Model file for the job. Use its own axes, mm. A direction names the side the tool comes from. Give positions to 0.01 mm unless a question says otherwise; leave off trailing zeros. Loops run counter-clockwise (first coordinate to the right, second up) from the corner with the lowest first, then second, coordinate; pieces in that order, holes last. Notation, with made-up numbers: (87, 80.5) - (109, 80.5) arc R32 ccw to (109, 117.5) - close; hole circle Ø1 at (60, 60). An arc over 180 degrees is marked (long way). Answer as CSV lines item,"result". Start each with the question number.
Item 1: Drill centre lines: L1, parallel to X at y = 8.5, z = 0; L2, parallel to X at y = -18, z = 0; L3, parallel to Z at x = 25, y = 5.5. Where is each one in solid material? Low to high. Write a range as from..to.
Item 2: Saw through at B-B on x = 44. Give the cut face in (y, z).
Item 3: Saw through at D-D on y = 24. Give the cut face in (x, z), plus the area to 3 significant figures.
Item 4: Saw through at C-C on z = 39.5. Give the cut face in (x, y).
Item 5: Pull direction Y, two halves, no side cores. Call faces 5 (the conical face through (-31.429, 39.806, -6.979)), 6 (the cylindrical face through (-19.297, 8.112, 35.157)), 7 (the flat face through (0, 0, 0)), 8 (the flat face through (-23, 16, 23)): pulls with the +Y half, pulls with the -Y half, needs draft (parallel to the pull), parting line crosses it, or undercut.
Item 6: Pin check, flat tips, straight feed: pin 1 (1 mm diameter, centred on x = 40, z = 3, fed in from -Y); pin 2 (9 mm diameter, centred on x = -22, z = 38.11, fed in from +Y); pin 3 (1 mm diameter, centred on x = -9.5, z = 32, fed in from +Y). Stop position of each tip, or through.
Item 7: Tool access for faces 1 (the cylindrical face through (25.966, 8.112, -38.626)), 2 (the cylindrical face through (10.81, -16.17, 34.34)), 3 (the cylindrical face through (7.21, 27.83, 22.89)), 4 (the flat face through (33, 0, 0)): list every direction of +Z, -Z, +X, -X, +Y, -Y with a clear straight run to the whole face (end or side of a thin tool).
Item 8: Saw through at A-A on y = 2. Give the cut face in (x, z).
from build123d import *

# Parameters (mm, degrees)
Y_KSEKLIK_EKSTR_ZYON1_DEPTH      = 40
Y_KSEKLIK_EKSTR_ZYON1_DEPTH_BACK = 32
IZIM1_R                          = 36
IZIM1_R_2                        = 24
IZIM1_3_R                        = 54
Y_KSEKLIK_EKSTR_ZYON2_DEPTH      = 16
PAH1_SIZE                        = 4
PAH3_SIZE                        = 4
IZIM6_R                          = 4
KES_EKSTR_ZYON1_DEPTH            = 16


with BuildPart() as part:
    # izim1 → Y_kseklik-Ekstr_zyon1 (new, two sides: drawn at the far end of the back side and taken through both)
    with BuildSketch(Plane(origin=(0, 0, 0), x_dir=(1, 0, 0), z_dir=(0, 1, 0)).offset(-Y_KSEKLIK_EKSTR_ZYON1_DEPTH_BACK)):
        with Locations(Location((0, 0, 0), (0, 0, 270))):
            Circle(IZIM1_R)
        with Locations(Location((0, 0, 0), (0, 0, 270))):
            Circle(IZIM1_R_2, mode=Mode.SUBTRACT)
    extrude(amount=Y_KSEKLIK_EKSTR_ZYON1_DEPTH + Y_KSEKLIK_EKSTR_ZYON1_DEPTH_BACK)

    # izim1_3 → Y_kseklik-Ekstr_zyon2 (add)
    with BuildSketch(Plane(origin=(0, 0, 0), x_dir=(1, 0, 0), z_dir=(0, 1, 0))):
        with Locations(Location((0, 0, 0), (0, 0, 270))):
            Circle(IZIM1_3_R)
    extrude(amount=Y_KSEKLIK_EKSTR_ZYON2_DEPTH)

    # Pah1
    pah1_edges = [part.edges().sort_by_distance(p)[0] for p in [
        (0, 40, -36),
    ]]
    chamfer(pah1_edges, length=PAH1_SIZE)

    # Pah3
    pah3_edges = [part.edges().sort_by_distance(p)[0] for p in [
        (0, -32, -36),
    ]]
    chamfer(pah3_edges, length=PAH3_SIZE)

    # Kes-S_p_r1: sweep along a curve in space
    with BuildLine() as kes_s_p_r1_path:
        ThreePointArc((0, 16, 36), (25.455844123, 16, 25.455844123), (36, 16, 0))
        ThreePointArc((36, 16, 0), (25.455844123, 16, -25.455844123), (0, 16, -36))
        ThreePointArc((0, 16, -36), (-25.455844123, 16, -25.455844123), (-36, 16, 0))
        ThreePointArc((-36, 16, 0), (-25.455844123, 16, 25.455844123), (0, 16, 36))
    # izim4 → Kes-S_p_r1 (sweep, cut)
    with BuildSketch(Plane(origin=(0, 0, 0), x_dir=(0, 0, -1), z_dir=(1, 0, 0))):
        with BuildLine():
            Line((-36, 20), (-36, 16))
            Line((-36, 16), (-32, 16))
            ThreePointArc((-32, 16), (-33.171572875, 18.828427125), (-36, 20))
        make_face()
    sweep(path=kes_s_p_r1_path.line, mode=Mode.SUBTRACT)

    # Kes-S_p_r3: sweep along a curve in space
    with BuildLine() as kes_s_p_r3_path:
        ThreePointArc((0, 0, 36), (25.455844123, 0, 25.455844123), (36, 0, 0))
        ThreePointArc((36, 0, 0), (25.455844123, 0, -25.455844123), (0, 0, -36))
        ThreePointArc((0, 0, -36), (-25.455844123, 0, -25.455844123), (-36, 0, 0))
        ThreePointArc((-36, 0, 0), (-25.455844123, 0, 25.455844123), (0, 0, 36))
    # izim5 → Kes-S_p_r3 (sweep, cut)
    with BuildSketch(Plane(origin=(0, 0, 0), x_dir=(0, 0, -1), z_dir=(1, 0, 0))):
        with BuildLine():
            Line((-36, 0), (-36, -4))
            ThreePointArc((-36, -4), (-33.171572875, -2.828427125), (-32, 0))
            Line((-32, 0), (-36, 0))
        make_face()
    sweep(path=kes_s_p_r3_path.line, mode=Mode.SUBTRACT)

    # izim6 → Kes-Ekstr_zyon1 (cut)
    with BuildSketch(Plane(origin=(0, 16, 0), x_dir=(1, 0, 0), z_dir=(0, 1, 0))):
        with Locations(Location((-22, 38.105117767, 0), (0, 0, 270))):
            Circle(IZIM6_R)
        with Locations(Location((22, 38.105117767, 0), (0, 0, 270))):
            Circle(IZIM6_R)
        with Locations(Location((44, 0, 0), (0, 0, 270))):
            Circle(IZIM6_R)
        with Locations(Location((22, -38.105117767, 0), (0, 0, 270))):
            Circle(IZIM6_R)
        with Locations(Location((-22, -38.105117767, 0), (0, 0, 270))):
            Circle(IZIM6_R)
        with Locations(Location((-44, 0, 0), (0, 0, 270))):
            Circle(IZIM6_R)
    extrude(amount=-KES_EKSTR_ZYON1_DEPTH, mode=Mode.SUBTRACT)


solid = part.part
Responses:
1,L1,"-54..-48, -40..40, 48..54"
1,L2,"-36..-24, 24..36"
1,L3,"-47.86..-40.75, -35.46..35.46, 40.75..47.86"
2,outline,"(0, -31.3) - (16, -31.3) - (16, -4) - (0, -4) - close; (0, 4) - (16, 4) - (16, 31.3) - (0, 31.3) - close"
3,outline,"circle Ø72 at (0, 0); hole circle Ø48 at (0, 0)"
3,area,"2,260 mm2"
4,outline,"(-36.82, 0) - (-25.75, 0) - (-25.75, 16) - (-36.82, 16) - close; (-18.25, 0) - (18.25, 0) - (18.25, 16) - (-18.25, 16) - close; (25.75, 0) - (36.82, 0) - (36.82, 16) - (25.75, 16) - close"
5,face 5,"pulls with the +Y half"
5,face 6,"needs draft"
5,face 7,"pulls with the -Y half"
5,face 8,"undercut"
6,pin 1,"y = 0"
6,pin 2,"y = 16"
6,pin 3,"y = 39.12"
7,face 1,"+Y, -Y"
7,face 2,"-Y"
7,face 3,"+Y"
7,face 4,"none"
8,outline,"circle Ø108 at (0, 0); hole circle Ø8 at (-44, 0); hole circle Ø8 at (-22, -38.11); hole circle Ø8 at (-22, 38.11); hole circle Ø8 at (22, -38.11); hole circle Ø8 at (22, 38.11); hole circle Ø8 at (44, 0)"
